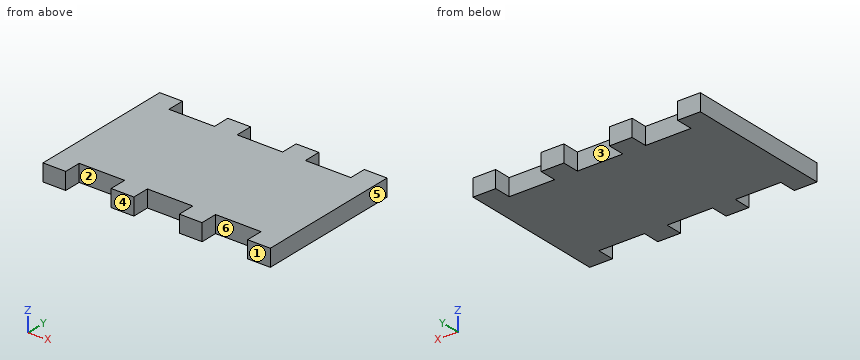
from build123d import *

# Parameters (mm, degrees)
ESQUISSE1_W        = 8
ESQUISSE1_H        = 6
BOSS_EXTRU_1_DEPTH = 6


with BuildPart() as part:
    # Esquisse1 → Boss.-Extru.1 (new body)
    with BuildSketch(Plane.XY):
        with Locations((4, -3)):
            Rectangle(ESQUISSE1_W, ESQUISSE1_H)
        with Locations((28, -3)):
            Rectangle(ESQUISSE1_W, ESQUISSE1_H)
        with Locations((52, -3)):
            Rectangle(ESQUISSE1_W, ESQUISSE1_H)
        Polygon((80, 20), (0, 20), (0, 0), (8, 0), (24, 0), (32, 0), (48, 0), (56, 0), (72, 0), (80, 0), align=None)
        Polygon((0, 40), (0, 20), (80, 20), (80, 40), (72, 40), (56, 40), (48, 40), (32, 40), (24, 40), (8, 40), align=None)
        with Locations((76, 43)):
            Rectangle(ESQUISSE1_W, ESQUISSE1_H)
        with Locations((52, 43)):
            Rectangle(ESQUISSE1_W, ESQUISSE1_H)
        with Locations((28, 43)):
            Rectangle(ESQUISSE1_W, ESQUISSE1_H)
        with Locations((4, 43)):
            Rectangle(ESQUISSE1_W, ESQUISSE1_H)
        with Locations((76, -3)):
            Rectangle(ESQUISSE1_W, ESQUISSE1_H)
    extrude(amount=BOSS_EXTRU_1_DEPTH)


solid = part.part
The model under review builds one solid part; all positions refer to its coordinate system, in mm. Face numbers are marked on the shaded views. A direction names the side the tool comes from. Round coordinates to 2 decimals unless told otherwise and drop trailing zeros. Write each loop counter-clockwise with the first axis right and the second up, starting at its lowest first coordinate (ties: lowest second). Pieces come first, ordered by that corner, then holes. Notation, with made-up numbers: M 0,10.25 L 30,10.25 A8 cw 30,17.25 Z; hole C -30,87.5 d10. An arc over 180 degrees is marked long. Answer as CSV lines item,"result". Start each with the question number.
Q1. The part is to be moulded in two halves that separate along X. For the marked faces 4, 5 and 6, say which applies: +X half, -X half, draft (parallel to the pull), parting line (faces both ways), or undercut.
Q2. Consider section B-B, the plane x = 16. Give the boundary of the cut face in (y, z).
Q3. Clearance check with flat-ended pins moving along their axes: P1, Ø1.8, axis at y = 44.5, z = 2.5, coming from the -X side; P2, Ø3, axis at x = 38, z = 3.5, coming from the +Y side; P3, Ø1, axis at x = 23, z = 5, coming from the -Y side. State where each tip first meets the part, or that it passes through.
Q4. Tool access review of the marked faces 1, 2 and 3: name each direction out of +Z, -Z, +X, -X, +Y, -Y from which nothing blocks a thin tool from reaching the whole face with its end or side.
Q5. Consider section A-A, the plane z = 0.9. Give the boundary of the cut face in (x, y), then the cut area to 3 significant figures.
Q6. Wall thickness on line 1 along X through (y, z) = (42.5, 4.4); line 2 along Y through (x, z) = (23, 1): over which ranges is each line inside the solid? List them lowest first.
Result set:
1,face 4,"draft"
1,face 5,"+X half"
1,face 6,"undercut"
2,outline,"M 0,0 L 40,0 L 40,6 L 0,6 Z"
3,P1,"stops at x = 0"
3,P2,"stops at y = 40"
3,P3,"stops at y = 0"
4,face 1,"+Z, -Z, +X, -X, -Y"
4,face 2,"+Z, -Z, -Y"
4,face 3,"+Z, -Z, +Y"
5,outline,"M 0,-6 L 8,-6 L 8,0 L 24,0 L 24,-6 L 32,-6 L 32,0 L 48,0 L 48,-6 L 56,-6 L 56,0 L 72,0 L 72,-6 L 80,-6 L 80,46 L 72,46 L 72,40 L 56,40 L 56,46 L 48,46 L 48,40 L 32,40 L 32,46 L 24,46 L 24,40 L 8,40 L 8,46 L 0,46 Z"
5,area,"3,580 mm²"
6,line 1,"x = 0 to 8, 24 to 32, 48 to 56, 72 to 80"
6,line 2,"y = 0 to 40"
